For this review, use the dimensioned drawing (mm, ordinates from the lowest corner) and the shaded views. A direction names the side the tool comes from. Give positions to 0.01 mm unless a question says otherwise; leave off trailing zeros. Order: outer loops, then holes, each group sorted by start corner. A loop starts at its lowest first (then second) coordinate and runs counter-clockwise, first axis right, second up. Notation, with made-up numbers: (33, -2) -> (92, -2) arc R12 cw to (92, 11) -> close; hole circle Ø10 at (53.25, 78.25). An arc over 180 degrees is marked (long way). Return JSON: item names as keys, results as strings.
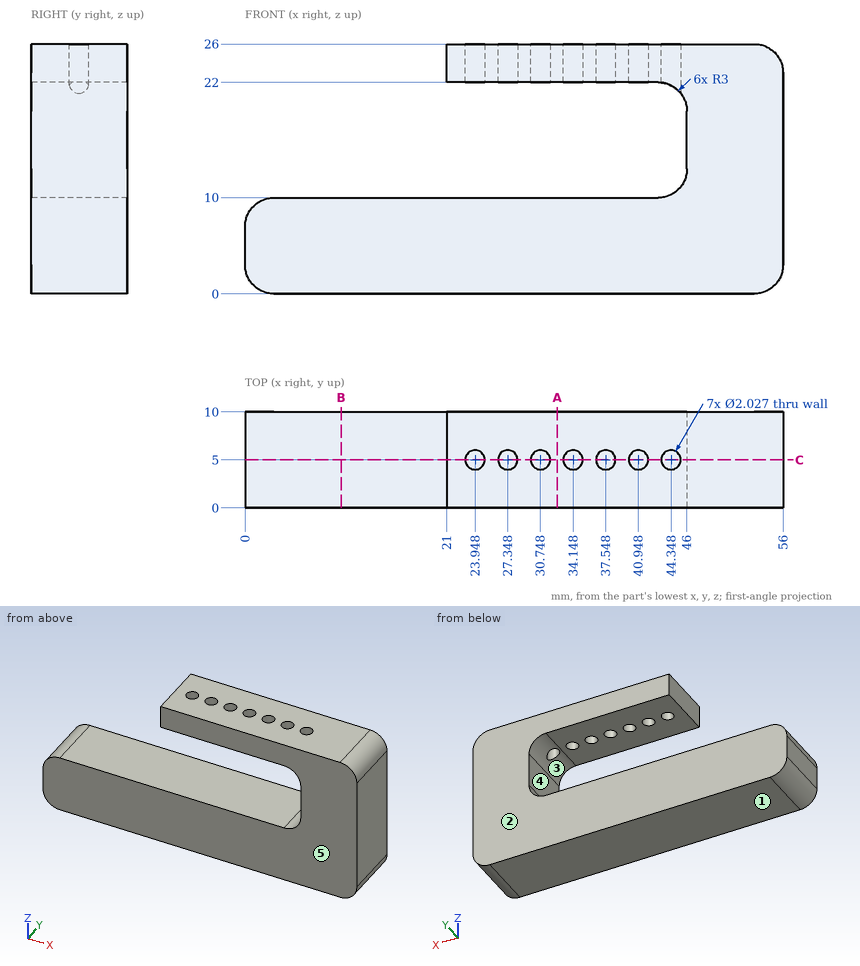
Item 1: Add section C-C (y = 5). Give the number of separate pieces and of enclosed holes in the cut face.
Result set:
{"separate pieces": "8", "enclosed holes": "0"}
Item 2: Machinability: for the marked faces 4 and 5, which of the approach directions +Z, -Z, +X, -X, +Y, -Y give a long, thin tool a straight path to every point of the face, cutting with its end or side? Answer none if there is none.
Result set:
{"face 4": "-X, +Y, -Y", "face 5": "+Z, -Z, +X, -X, -Y"}
Item 3: Add section A-A (x = 32.5). Give the boundary of the cut face in (y, z).
Result set:
{"outline": "(0, 0) -> (10, 0) -> (10, 10) -> (0, 10) -> close; (0, 22) -> (10, 22) -> (10, 26) -> (0, 26) -> close"}
Item 4: Add section B-B (x = 10). Give the boundary of the cut face in (y, z).
Result set:
{"outline": "(0, 0) -> (10, 0) -> (10, 10) -> (0, 10) -> close"}
Item 5: Wall thickness on L1, parallel to Z at x = 26, y = 9.5; L2, parallel to Z at x = 37, y = 5; L3, parallel to X at y = 5.25, z = 18.25: over which ranges is each line inside the solid? List them lowest first. Write a range as [from, to].
Result set:
{"L1": "z = [0, 10], [22, 26]", "L2": "z = [0, 10]", "L3": "x = [46, 56]"}
Item 6: Mouldability with a two-part tool opening along Z and no side actions: class the marked faces 1, 2 and 3 as released by +Z, released by -Z, zero draft, split by the parting line, or undercut.
Result set:
{"face 1": "released by -Z", "face 2": "zero draft", "face 3": "undercut"}
Item 7: For pin 1 (1.5 mm diameter, centred on y = 5, z = 18.5, fed in from -X); pin 2 (1.8 mm diameter, centred on x = 23.95, y = 5, fed in from +Z); pin 3 (4 mm diameter, centred on y = 4.5, z = 13, fed in from -X), all flat-tipped, find the tip position at first contact; note any pin that passes through.
Result set:
{"pin 1": "stops at x = 45.99", "pin 2": "stops at z = 10", "pin 3": "stops at x = 45.24"}
